Autodesk Inventor part; units mm, degrees
ref_plane "ip_st_ir_1_1_XY" through (1.5, 4, 0) normal (1, 0, 0) x (0, 0, -1)
ref_plane "ip_st_ir_1_1_YZ" through (1.5, 4, 0) normal (0, 0, -1) x (0, 1, 0)
ref_plane "ip_st_ir_1_1_ZX" through (1.5, 4, 0) normal (0, 1, 0) x (1, 0, 0)
sketch "Sketch_1" plane through (0, 0, 0) normal (0, 0, 1) x (1, 0, 0)
  line L0 (3, 0) -> (0, 0)
  arc A0 (0, 3.1) -> (0.1, 3) centre (0.1, 3.1) ccw
  line L1 (0.1, 3) -> (2.9, 3)
  arc A1 (2.9, 3) -> (3, 3.1) centre (2.9, 3.1) ccw
  line L2 (3, 3.1) -> (3, 3.52)
  line L3 (3, 3.52) -> (1.86, 3.52)
  arc A2 (1.14, 3.52) -> (1.86, 3.52) centre (1.5, 4) ccw
  line L4 (1.14, 3.52) -> (0, 3.52)
  line L5 (0, 3.52) -> (0, 3.1)
revolve "Revolution1" add sketch "Sketch_1" angle 360 about axis through (3, 0, 0) along (1, 0, 0)
ref_plane "ip_st_ir_1_1_XY" through (1.5, 4, 0) normal (1, 0, 0) x (0, 0, -1)
ref_plane "ip_st_ir_1_1_YZ" through (1.5, 4, 0) normal (0, 0, -1) x (0, 1, 0)
ref_plane "ip_st_ir_1_1_ZX" through (1.5, 4, 0) normal (0, 1, 0) x (1, 0, 0)
ref_plane "ip_st_ir_1_10_XY" through (1.5, -3.6955, -1.5307) normal (1, 0, 0) x (0, 0, -1)
ref_plane "ip_st_ir_1_10_YZ" through (1.5, -3.6955, -1.5307) normal (0, 0, -1) x (0, 1, 0)
ref_plane "ip_st_ir_1_10_ZX" through (1.5, -3.6955, -1.5307) normal (0, 1, 0) x (1, 0, 0)
ref_plane "ip_st_ir_1_11_XY" through (1.5, -2.8284, -2.8284) normal (1, 0, 0) x (0, 0, -1)
ref_plane "ip_st_ir_1_11_YZ" through (1.5, -2.8284, -2.8284) normal (0, 0, -1) x (0, 1, 0)
ref_plane "ip_st_ir_1_11_ZX" through (1.5, -2.8284, -2.8284) normal (0, 1, 0) x (1, 0, 0)
ref_plane "ip_st_ir_1_12_XY" through (1.5, -1.5307, -3.6955) normal (1, 0, 0) x (0, 0, -1)
ref_plane "ip_st_ir_1_12_YZ" through (1.5, -1.5307, -3.6955) normal (0, 0, -1) x (0, 1, 0)
ref_plane "ip_st_ir_1_12_ZX" through (1.5, -1.5307, -3.6955) normal (0, 1, 0) x (1, 0, 0)
ref_plane "ip_st_ir_1_13_XY" through (1.5, 0, -4) normal (1, 0, 0) x (0, 0, -1)
ref_plane "ip_st_ir_1_13_YZ" through (1.5, 0, -4) normal (0, 0, -1) x (0, 1, 0)
ref_plane "ip_st_ir_1_13_ZX" through (1.5, 0, -4) normal (0, 1, 0) x (1, 0, 0)
ref_plane "ip_st_ir_1_14_XY" through (1.5, 1.5307, -3.6955) normal (1, 0, 0) x (0, 0, -1)
ref_plane "ip_st_ir_1_14_YZ" through (1.5, 1.5307, -3.6955) normal (0, 0, -1) x (0, 1, 0)
ref_plane "ip_st_ir_1_14_ZX" through (1.5, 1.5307, -3.6955) normal (0, 1, 0) x (1, 0, 0)
ref_plane "ip_st_ir_1_15_XY" through (1.5, 2.8284, -2.8284) normal (1, 0, 0) x (0, 0, -1)
ref_plane "ip_st_ir_1_15_YZ" through (1.5, 2.8284, -2.8284) normal (0, 0, -1) x (0, 1, 0)
ref_plane "ip_st_ir_1_15_ZX" through (1.5, 2.8284, -2.8284) normal (0, 1, 0) x (1, 0, 0)
ref_plane "ip_st_ir_1_16_XY" through (1.5, 3.6955, -1.5307) normal (1, 0, 0) x (0, 0, -1)
ref_plane "ip_st_ir_1_16_YZ" through (1.5, 3.6955, -1.5307) normal (0, 0, -1) x (0, 1, 0)
ref_plane "ip_st_ir_1_16_ZX" through (1.5, 3.6955, -1.5307) normal (0, 1, 0) x (1, 0, 0)
ref_plane "ip_st_ir_1_2_XY" through (1.5, 3.6955, 1.5307) normal (1, 0, 0) x (0, 0, -1)
ref_plane "ip_st_ir_1_2_YZ" through (1.5, 3.6955, 1.5307) normal (0, 0, -1) x (0, 1, 0)
ref_plane "ip_st_ir_1_2_ZX" through (1.5, 3.6955, 1.5307) normal (0, 1, 0) x (1, 0, 0)
ref_plane "ip_st_ir_1_3_XY" through (1.5, 2.8284, 2.8284) normal (1, 0, 0) x (0, 0, -1)
ref_plane "ip_st_ir_1_3_YZ" through (1.5, 2.8284, 2.8284) normal (0, 0, -1) x (0, 1, 0)
ref_plane "ip_st_ir_1_3_ZX" through (1.5, 2.8284, 2.8284) normal (0, 1, 0) x (1, 0, 0)
ref_plane "ip_st_ir_1_4_XY" through (1.5, 1.5307, 3.6955) normal (1, 0, 0) x (0, 0, -1)
ref_plane "ip_st_ir_1_4_YZ" through (1.5, 1.5307, 3.6955) normal (0, 0, -1) x (0, 1, 0)
ref_plane "ip_st_ir_1_4_ZX" through (1.5, 1.5307, 3.6955) normal (0, 1, 0) x (1, 0, 0)
ref_plane "ip_st_ir_1_5_XY" through (1.5, 0, 4) normal (1, 0, 0) x (0, 0, -1)
ref_plane "ip_st_ir_1_5_YZ" through (1.5, 0, 4) normal (0, 0, -1) x (0, 1, 0)
ref_plane "ip_st_ir_1_5_ZX" through (1.5, 0, 4) normal (0, 1, 0) x (1, 0, 0)
ref_plane "ip_st_ir_1_6_XY" through (1.5, -1.5307, 3.6955) normal (1, 0, 0) x (0, 0, -1)
ref_plane "ip_st_ir_1_6_YZ" through (1.5, -1.5307, 3.6955) normal (0, 0, -1) x (0, 1, 0)
ref_plane "ip_st_ir_1_6_ZX" through (1.5, -1.5307, 3.6955) normal (0, 1, 0) x (1, 0, 0)
ref_plane "ip_st_ir_1_7_XY" through (1.5, -2.8284, 2.8284) normal (1, 0, 0) x (0, 0, -1)
ref_plane "ip_st_ir_1_7_YZ" through (1.5, -2.8284, 2.8284) normal (0, 0, -1) x (0, 1, 0)
ref_plane "ip_st_ir_1_7_ZX" through (1.5, -2.8284, 2.8284) normal (0, 1, 0) x (1, 0, 0)
ref_plane "ip_st_ir_1_8_XY" through (1.5, -3.6955, 1.5307) normal (1, 0, 0) x (0, 0, -1)
ref_plane "ip_st_ir_1_8_YZ" through (1.5, -3.6955, 1.5307) normal (0, 0, -1) x (0, 1, 0)
ref_plane "ip_st_ir_1_8_ZX" through (1.5, -3.6955, 1.5307) normal (0, 1, 0) x (1, 0, 0)
ref_plane "ip_st_ir_1_9_XY" through (1.5, -4, 0) normal (1, 0, 0) x (0, 0, -1)
ref_plane "ip_st_ir_1_9_YZ" through (1.5, -4, 0) normal (0, 0, -1) x (0, 1, 0)
ref_plane "ip_st_ir_1_9_ZX" through (1.5, -4, 0) normal (0, 1, 0) x (1, 0, 0)
ref_plane "ip_st_ir_1a_XY" through (0, 0, 0) normal (1, 0, 0) x (0, 0, -1)
ref_plane "ip_st_ir_1a_YZ" through (0, 0, 0) normal (0, 0, -1) x (0, 1, 0)
ref_plane "ip_st_ir_1a_ZX" through (0, 0, 0) normal (0, 1, 0) x (1, 0, 0)
ref_plane "ip_st_ir_2a_XY" through (0.1992, 0, 0) normal (1, 0, 0) x (0, 0, -1)
ref_plane "ip_st_ir_2a_YZ" through (0.1992, 0, 0) normal (0, 0, -1) x (0, 1, 0)
ref_plane "ip_st_ir_2a_ZX" through (0.1992, 0, 0) normal (0, 1, 0) x (1, 0, 0)
properties part number "MR106ZZ1 Inner Ring"
Check sheet for the modelled part. Datum: model origin and axes. Units: mm. Coordinates: 2 decimals unless noted, no trailing zeros. Loops run counter-clockwise (first coordinate to the right, second up) from the corner with the lowest first, then second, coordinate; pieces in that order, holes last. Notation, with made-up numbers: (18, 51.5) -> (66, 51.5) arc R33 cw to (66, 82.5) -> close; hole circle Ø10 at (-30, 58). An arc over 180 degrees is marked (long way). Answer in a Markdown table with one row per item.
1. Sectioned sample at A-A, the plane y = 0. Record the boundary of the cut face in (x, z).
Check values:
| item | result |
|---|---|
| outline | (0, -3.52) -> (1.14, -3.52) arc R0.6 cw to (1.86, -3.52) -> (3, -3.52) -> (3, -3.1) arc R0.1 ccw to (2.9, -3) -> (0.1, -3) arc R0.1 ccw to (0, -3.1) -> close; (0, 3.1) arc R0.1 ccw to (0.1, 3) -> (2.9, 3) arc R0.1 ccw to (3, 3.1) -> (3, 3.52) -> (1.86, 3.52) arc R0.6 cw to (1.14, 3.52) -> (0, 3.52) -> close |
2. Sectioned sample at C-C, the plane x = 2.25. Record the boundary of the cut face in (y, z), then the cut area to 3 significant figures.
Check values:
| item | result |
|---|---|
| outline | circle Ø7.04 at (0, 0); hole circle Ø6 at (0, 0) |
| area | 10.7 mm2 |
3. Material ranges on line 1 along Z through (x, y) = (2.25, 0); line 2 along Y through (x, z) = (0.8, 0.25); line 3 along Z through (x, y) = (1.6, 0), recorded low to high. Write a range as [from, to].
Check values:
| item | result |
|---|---|
| line 1 | z = [-3.52, -3], [3, 3.52] |
| line 2 | y = [-3.51, -2.99], [2.99, 3.51] |
| line 3 | z = [-3.41, -3], [3, 3.41] |
4. Sectioned sample at D-D, the plane x = 1.75. Record the boundary of the cut face in (y, z), then the cut area to 3 significant figures.
Check values:
| item | result |
|---|---|
| outline | circle Ø6.91 at (0, 0); hole circle Ø6 at (0, 0) |
| area | 9.22 mm2 |
5. Release check for a two-part mould opening along Z. For faces 1 (the face through (2.422, -0.763, 3.436)), 2 (the face through (2, -3, 0)) record: released by +Z, released by -Z, zero draft, split by the parting line, or undercut.
Check values:
| item | result |
|---|---|
| face 1 | split by the parting line |
| face 2 | undercut |
